```python
from build123d import *

# Parameters (mm, degrees)
SKETCH1_R           = 6.35
BOSS_EXTRUDE1_DEPTH = 6.35


with BuildPart() as part:
    # Sketch1 → Boss-Extrude1 (new body)
    with BuildSketch(Plane.XY):
        with BuildLine():
            Line((-13.335, 0), (-13.335, -5.715))
            ThreePointArc((-13.335, -5.715), (-14.26493597, -7.96006403), (-16.51, -8.89))
            Line((-16.51, -8.89), (-16.51, -19.05))
            Line((-16.51, -19.05), (-10.4394, -19.05))
            ThreePointArc((-10.4394, -19.05), (-8.242182532, -13.745447789), (-2.93763032, -11.54823032))
            Line((-2.93763032, -11.54823032), (2.93763032, -11.54823032))
            ThreePointArc((2.93763032, -11.54823032), (8.242182532, -13.745447789), (10.4394, -19.05))
            Line((10.4394, -19.05), (16.51, -19.05))
            Line((16.51, -19.05), (16.51, -8.89))
            ThreePointArc((16.51, -8.89), (14.26493597, -7.96006403), (13.335, -5.715))
            Line((13.335, -5.715), (13.335, 0))
            ThreePointArc((13.335, 0), (0, 13.335), (-13.335, 0))
        make_face()
        Circle(SKETCH1_R, mode=Mode.SUBTRACT)
    extrude(amount=BOSS_EXTRUDE1_DEPTH)

    # Sketch2 → Tap Drill for #6-32 Tap1 (revolve, cut)
    with BuildSketch(Plane(origin=(-13.4747, -19.05, 3.175), x_dir=(0, 0, -1), z_dir=(1, 0, 0))):
        Polygon((0, 0), (0, 8.43269403), (1.35255, 7.62), (1.35255, 0), align=None)
    tap_drill_for_6_32_tap1 = revolve(axis=Axis((-13.4747, -25.4, 3.175), (0, 1, 0)), mode=Mode.SUBTRACT)

    # Mirror1: Tap Drill for #6-32 Tap1 across plane
    add(tap_drill_for_6_32_tap1.mirror(Plane(origin=(0, 0, 0), x_dir=(0, 0, 1), z_dir=(1, 0, 0))), mode=Mode.SUBTRACT)


solid = part.part
```
Design review of the part built by this model. Coordinates are the model's own, in mm. A direction names the side the tool comes from. Coordinates: 2 decimals unless noted, no trailing zeros. Write each loop counter-clockwise with the first axis right and the second up, starting at its lowest first coordinate (ties: lowest second). Pieces come first, ordered by that corner, then holes. Notation, with made-up numbers: M 52.25,-31.5 L 87.25,-31.5 A11 cw 87.25,-13.5 Z; hole C 64,68 d2. An arc over 180 degrees is marked long. Answer as a JSON object with one key per item and string values.
Item 1: Add section C-C, the plane y = 9. Give the boundary of the cut face in (x, z), and give its area (3 significant figures).
Outcome:
{"outline": "M -9.84,0 L 9.84,0 L 9.84,6.35 L -9.84,6.35 Z", "area": "125 mm²"}
Item 2: Add section B-B, the plane y = 2. Give the boundary of the cut face in (x, z), and give its area (3 significant figures).
Outcome:
{"outline": "M -13.18,0 L -6.03,0 L -6.03,6.35 L -13.18,6.35 Z; M 6.03,0 L 13.18,0 L 13.18,6.35 L 6.03,6.35 Z", "area": "90.9 mm²"}
Item 3: Wall thickness on probe 1 along X at (y, z) = (-13, 3); probe 2 along X at (y, z) = (4, 3); probe 3 along Y at (x, z) = (2, 1.25): over which ranges is each line inside the solid? List them lowest first.
Outcome:
{"probe 1": "-16.51 to -14.82, -12.13 to -7.37, 7.37 to 12.13, 14.82 to 16.51", "probe 2": "-12.72 to -4.93, 4.93 to 12.72", "probe 3": "-11.55 to -6.03, 6.03 to 13.18"}
Item 4: Add section A-A, the plane x = 0. Give the boundary of the cut face in (y, z) (3 decimals), and give its area (3 significant figures).
Outcome:
{"outline": "M -11.548,0 L -6.35,0 L -6.35,6.35 L -11.548,6.35 Z; M 6.35,0 L 13.335,0 L 13.335,6.35 L 6.35,6.35 Z", "area": "77.4 mm²"}
Item 5: Add section D-D, the plane x = -11. Give the boundary of the cut face in (y, z).
Outcome:
{"outline": "M -19.05,0 L 7.54,0 L 7.54,6.35 L -19.05,6.35 Z"}
Item 6: Draft analysis for pull direction Y (two halves, no side actions). For faces 1 (the cylindrical face through (-1.38, -6.2, 3.13)), 2 (the cylindrical face through (-8.3, -13.804, 3.131)), 3 (the flat face through (-16.51, -14, 3)), state which applies: pulls with the +Y half, pulls with the -Y half, needs draft (parallel to the pull), parting line crosses it, or undercut.
Outcome:
{"face 1": "undercut", "face 2": "pulls with the -Y half", "face 3": "needs draft"}
Item 7: Insertion check: pin 1 Ø1.7 at (y, z) = (-3.5, 4.5) entering from -X (3 decimals); pin 2 Ø10 at (x, y) = (0, 0) entering from -Z; pin 3 Ø1 at (y, z) = (4, 1) entering from +X; pin 4 Ø8 at (x, y) = (10, 0) entering from -Z. Each pin has a flat end and moves straight along its axis. Give the tip position at first contact, or say it passes through.
Outcome:
{"pin 1": "x = -13.335", "pin 2": "through", "pin 3": "x = 12.87", "pin 4": "z = 0"}
Item 8: Machinability: for faces 4 (the flat face through (13.335, -3, 3)), 5 (the flat face through (-13.335, -3, 3)), 6 (the cylindrical face through (14.816, -15.293, 3.351)), which of the approach directions +Z, -Z, +X, -X, +Y, -Y give a long, thin tool a straight path to every point of the face, cutting with its end or side? Answer none if there is none.
Outcome:
{"face 4": "+Z, -Z, +X, +Y", "face 5": "+Z, -Z, -X, +Y", "face 6": "-Y"}
